```python
from build123d import *


with BuildPart() as part:
    # Sketch1 → Revolve1 (revolve)
    with BuildSketch(Plane.XY):
        with BuildLine():
            Line((0, 0), (0, -33.42037452))
            Line((0, -33.42037452), (11.846734569, -33.42037452))
            Line((11.846734569, -33.42037452), (11.846734569, -7.708743439))
            ThreePointArc((11.846734569, -7.708743439), (11.605583733, -6.75666696), (10.940284949, -6.034184521))
            Line((10.940284949, -6.034184521), (6.829816905, -3.349893247))
            ThreePointArc((6.829816905, -3.349893247), (6.164518121, -2.627410808), (5.923367285, -1.67533433))
            Line((5.923367285, -1.67533433), (5.923367285, -1))
            ThreePointArc((5.923367285, -1), (5.630474066, -0.292893219), (4.923367285, 0))
            Line((4.923367285, 0), (0, 0))
        make_face()
    revolve(axis=Axis((0, 0, 0), (0, -1, 0)))


solid = part.part
```
Input: part model. Units: mm. Frame: model coordinates. A direction names the side the tool comes from. Round coordinates to 2 decimals unless told otherwise and drop trailing zeros. Loops run counter-clockwise (first coordinate to the right, second up) from the corner with the lowest first, then second, coordinate; pieces in that order, holes last.
1) Section query B-B on y = -10.5. Return the cut outline in (x, z), plus the area to 3 significant figures.
Ans:
outline: circle Ø23.69 at (0, 0)
area: 441 mm2
2) Material intervals for line 1 (Z direction, x = -8, y = -23); line 2 (Y direction, x = -4, z = -7.25); line 3 (Z direction, x = -2.5, y = -25), sorted ascending.
Ans:
line 1: z = -8.74 to 8.74
line 2: y = -33.42 to -4.3
line 3: z = -11.58 to 11.58
3) Pin query (flat end, axial travel): pin 1 (4 mm diameter, centred on x = 4, z = -8.5, fed in from +Y); pin 2 (8 mm diameter, centred on x = 9, y = -9.5, fed in from -Z); pin 3 (2 mm diameter, centred on y = -3.5, z = -9, fed in from +X); pin 4 (3 mm diameter, centred on y = -7, z = 7, fed in from +X). Return the tip coordinate at first contact, or that it passes through.
Ans:
pin 1: stops at y = -3.72
pin 2: stops at z = -10.74
pin 3: passes through
pin 4: stops at x = 10.44
4) Set-up query: faces 1 (the flat face through (0, 0, 0)), 2 (the cylindrical face through (-1.284, -1.333, -5.783)). Return all of +Z, -Z, +X, -X, +Y, -Y with unobstructed straight access to the full face (end or side cutting, diameter ignored); none if empty.
Ans:
face 1: +Z, -Z, +X, -X, +Y
face 2: +Y
5) Section query A-A on x = 0. Return the cut outline in (y, z).
Ans:
outline: (-33.42, -11.85) - (-7.71, -11.85) arc R2 ccw to (-6.03, -10.94) - (-3.35, -6.83) arc R2 cw to (-1.68, -5.92) - (-1, -5.92) arc R1 ccw to (0, -4.92) - (0, 4.92) arc R1 ccw to (-1, 5.92) - (-1.68, 5.92) arc R2 cw to (-3.35, 6.83) - (-6.03, 10.94) arc R2 ccw to (-7.71, 11.85) - (-33.42, 11.85) - close
